Part print with two shaded views. Sizes in mm from the minimum x, y, z corner. A direction names the side the tool comes from. Round coordinates to 2 decimals unless told otherwise and drop trailing zeros. Order: outer loops, then holes, each group sorted by start corner. A loop starts at its lowest first (then second) coordinate and runs counter-clockwise, first axis right, second up. Notation, with made-up numbers: M 74.5,1 L 88.5,1 A12 ccw 88.5,5 Z; hole C 74.25,56 d5. An arc over 180 degrees is marked long. Put each result on its own line as item: value.
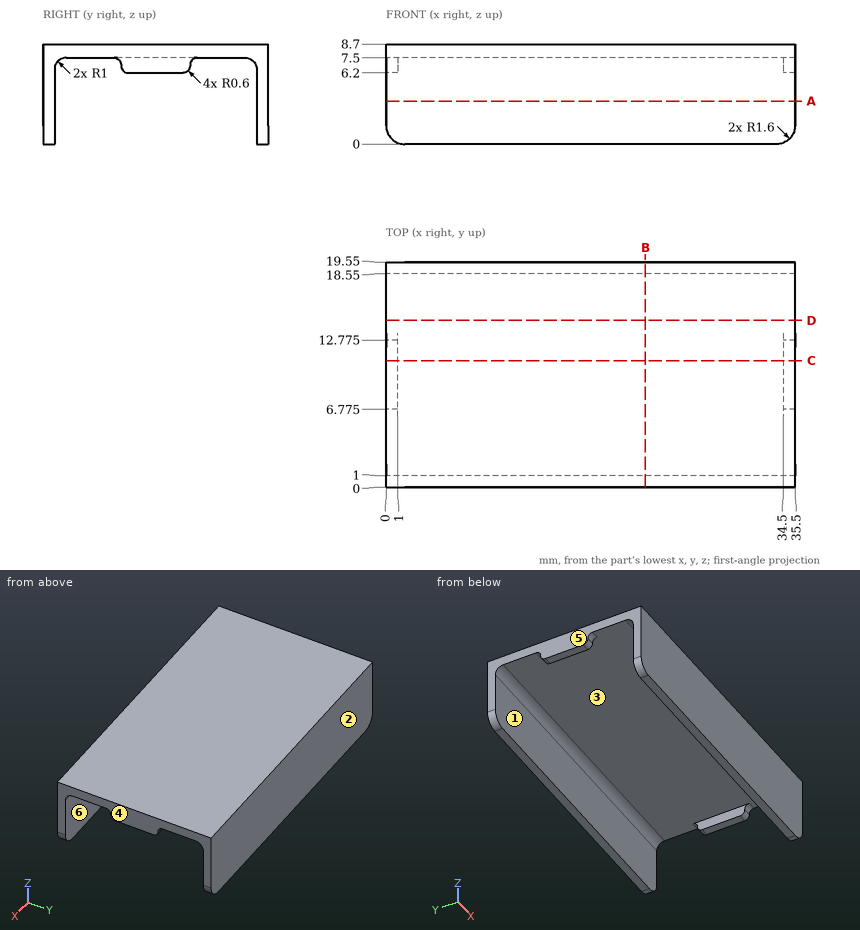
Item 1: Pin check, flat tips, straight feed: P1, Ø0.8, axis at x = 0.5, y = 10.5, coming from the -Z side; P2, Ø2, axis at x = 25.5, z = 7, coming from the -Y side. Stop position of each tip, or through.
Answers below:
P1: z = 6.2
P2: y = 0
Item 2: Band-saw the part on C-C on y = 11. Give the cut face in (x, z), and give its area (3 significant figures).
Answers below:
outline: M 0,6.2 L 1,6.2 L 1,7.5 L 34.5,7.5 L 34.5,6.2 L 35.5,6.2 L 35.5,8.7 L 0,8.7 Z
area: 45.2 mm²
Item 3: Mould opens along X. For the marked faces 3, 4, 5 and 6 say: pulls with the +X half, pulls with the -X half, needs draft (parallel to the pull), parting line crosses it, or undercut.
Answers below:
face 3: undercut
face 4: pulls with the +X half
face 5: pulls with the -X half
face 6: needs draft
Item 4: Tool access for the marked faces 1 and 2: list every direction of +Z, -Z, +X, -X, +Y, -Y with a clear straight run to the whole face (end or side of a thin tool).
Answers below:
face 1: -Z, +X, -X
face 2: +Z, -Z, +X, -X, +Y
Item 5: Band-saw the part on D-D on y = 14.5. Give the cut face in (x, z).
Answers below:
outline: M 0,7.5 L 35.5,7.5 L 35.5,8.7 L 0,8.7 Z
Item 6: Band-saw the part on A-A on z = 3.75. Give the cut face in (x, y), and give its area (3 significant figures).
Answers below:
outline: M 0,0 L 35.5,0 L 35.5,1 L 0,1 Z; M 0,18.55 L 35.5,18.55 L 35.5,19.55 L 0,19.55 Z
area: 71.0 mm²
Item 7: Probe line 1 along Y through (x, z) = (8, 4); line 2 along Z through (x, y) = (14, 8.5). List the from-to ranges inside material, lowest first. Write a range as [from, to].
Answers below:
line 1: [0, 1], [18.55, 19.55]
line 2: [7.5, 8.7]
Item 8: Band-saw the part on B-B on x = 22.5. Give the cut face in (y, z), and give its area (3 significant figures).
Answers below:
outline: M 0,0 L 1,0 L 1,6.5 A1 cw 2,7.5 L 17.55,7.5 A1 cw 18.55,6.5 L 18.55,0 L 19.55,0 L 19.55,8.7 L 0,8.7 Z
area: 38.9 mm²
